from build123d import *

# Parameters (mm, degrees)
ESQUISSE15_R        = 1.5
BOSS_EXTRU_15_DEPTH = 3


with BuildPart() as part:
    # Esquisse15 → Boss.-Extru.15 (new body)
    with BuildSketch(Plane.XY):
        with BuildLine():
            Line((198.647142503, 65.56420703), (126.393109195, 65.56420703))
            ThreePointArc((126.393109195, 65.56420703), (123.893109195, 65.881748664), (121.551880013, 66.81420703))
            ThreePointArc((121.551880013, 66.81420703), (112.647142503, 61.56420703), (121.551880013, 56.31420703))
            ThreePointArc((121.551880013, 56.31420703), (123.893109195, 57.246665395), (126.393109195, 57.56420703))
            Line((126.393109195, 57.56420703), (198.647142503, 57.56420703))
            ThreePointArc((198.647142503, 57.56420703), (202.647142503, 61.56420703), (198.647142503, 65.56420703))
        make_face()
        with Locations((118.647142503, 61.56420703)):
            Circle(ESQUISSE15_R, mode=Mode.SUBTRACT)
        with Locations((198.647142503, 61.56420703)):
            Circle(ESQUISSE15_R, mode=Mode.SUBTRACT)
    extrude(amount=BOSS_EXTRU_15_DEPTH)


solid = part.part
The model under review builds one solid part; all positions refer to its coordinate system, in mm. A direction names the side the tool comes from. Round coordinates to 2 decimals unless told otherwise and drop trailing zeros. Write each loop counter-clockwise with the first axis right and the second up, starting at its lowest first coordinate (ties: lowest second). Pieces come first, ordered by that corner, then holes. Notation, with made-up numbers: M 46.25,77 L 73.25,77 A15 ccw 73.25,101 Z; hole C 57.25,86 d1. An arc over 180 degrees is marked long. Use a Markdown table: item, result. Add a question column.
Q1. We need section B-B, the plane x = 196. State the section outline as (y, z) points.
Q2. To check wall thickness, follow line 1 (X direction, y = 61.5, z = 0.35); line 2 (X direction, y = 61.25, z = 0.65); line 3 (Y direction, x = 150, z = 0.95). State the ranges of each line that lie inside material, in increasing order.
Q3. We need section A-A, the plane z = 1.45. State the section outline as (x, y) points, plus the area to 3 significant figures.
Q4. The part is to be moulded in two halves that separate along Y. For faces 3 (the face through (157, 62, 0)), 4 (the face through (163, 65.564, 1)), 5 (the face through (120.08, 62.01, 1.48)), say which applies: pulls with the +Y half, pulls with the -Y half, needs draft (parallel to the pull), parting line crosses it, or undercut.
Q5. Machinability: for faces 1 (the face through (200.08, 62.01, 1.48)), 2 (the face through (162, 57.564, 1)), which of the approach directions +Z, -Z, +X, -X, +Y, -Y give a long, thin tool a straight path to every point of the face, cutting with its end or side? Answer none if there is none.
Q6. Insertion check: pin 1 (1.5 mm diameter, centred on x = 159.5, z = 1, fed in from +Y); pin 2 (0.9 mm diameter, centred on x = 145, z = 1, fed in from -Y). Each pin has a flat end and moves straight along its axis. Give the tip position at first contact, or say it passes through.
Q7. We need section C-C, the plane y = 59. State the section outline as (x, z) points, plus the area to 3 significant figures.
Findings below:
| question | item | result |
|---|---|---|
| 1 | outline | M 57.56,0 L 65.56,0 L 65.56,3 L 57.56,3 Z |
| 2 | line 1 | x = 112.65 to 117.15, 120.15 to 197.15, 200.15 to 202.65 |
| 2 | line 2 | x = 112.66 to 117.18, 120.11 to 197.18, 200.11 to 202.63 |
| 2 | line 3 | y = 57.56 to 65.56 |
| 3 | outline | M 121.55,56.31 A10 cw 126.39,57.56 L 198.65,57.56 A4 ccw 198.65,65.56 L 126.39,65.56 A10 cw 121.55,66.81 A6 ccw long Z; hole C 118.65,61.56 d3; hole C 198.65,61.56 d3 |
| 3 | area | 722 mm² |
| 4 | face 3 | needs draft |
| 4 | face 4 | pulls with the +Y half |
| 4 | face 5 | undercut |
| 5 | face 1 | +Z, -Z |
| 5 | face 2 | +Z, -Z, +X, -Y |
| 6 | pin 1 | stops at y = 65.56 |
| 6 | pin 2 | stops at y = 57.56 |
| 7 | outline | M 113.22,0 L 201.72,0 L 201.72,3 L 113.22,3 Z |
| 7 | area | 265 mm² |
